Part print with two shaded views. Sizes in mm from the minimum x, y, z corner. A direction names the side the tool comes from. Coordinates: 2 decimals unless noted, no trailing zeros. Write each loop counter-clockwise with the first axis right and the second up, starting at its lowest first coordinate (ties: lowest second). Pieces come first, ordered by that corner, then holes. Notation, with made-up numbers: (-1.75, 62) - (33.25, 62) arc R34 ccw to (33.25, 99) - close; hole circle Ø1 at (18, 77.25). An arc over 180 degrees is marked (long way). Answer in a Markdown table with one row per item. Add a question column.
Q1. Pin check, flat tips, straight feed: pin 1 (1 mm diameter, centred on y = 38.5, z = 2, fed in from -X); pin 2 (3 mm diameter, centred on y = 41.5, z = 9.5, fed in from +X); pin 3 (2 mm diameter, centred on x = 39, z = 6.5, fed in from +Y). Stop position of each tip, or through.
Q2. Two-plate mould, pull along X, no slides. Class the marked faces 3, 4 and 5: +X half, -X half, draft (parallel to the pull), parting line (faces both ways), or undercut.
Q3. Band-saw the part on A-A (y = 26). List the corners of the cut face in (x, z).
Q4. Band-saw the part on D-D (y = 46.5). List the corners of the cut face in (x, z), and give its area (3 significant figures).
Q5. Drill centre lines: line 1 along Z through (x, y) = (23, 49); line 2 along X through (y, z) = (25, 3.25); line 3 along Z through (x, y) = (24, 47). Where is each one in solid material? Low to high. Write a range as from..to.
Q6. Band-saw the part on C-C (z = 2.25). List the corners of the cut face in (x, y), and give its area (3 significant figures).
Q7. 3-axis set-ups, long thin cutter, end or side, ignore diameter. For the marked faces 1 and 2: which of +Z, -Z, +X, -X, +Y, -Y reach the whole face in a straight line?
Q8. Band-saw the part on B-B (x = 23). List the corners of the cut face in (y, z), and give its area (3 significant figures).
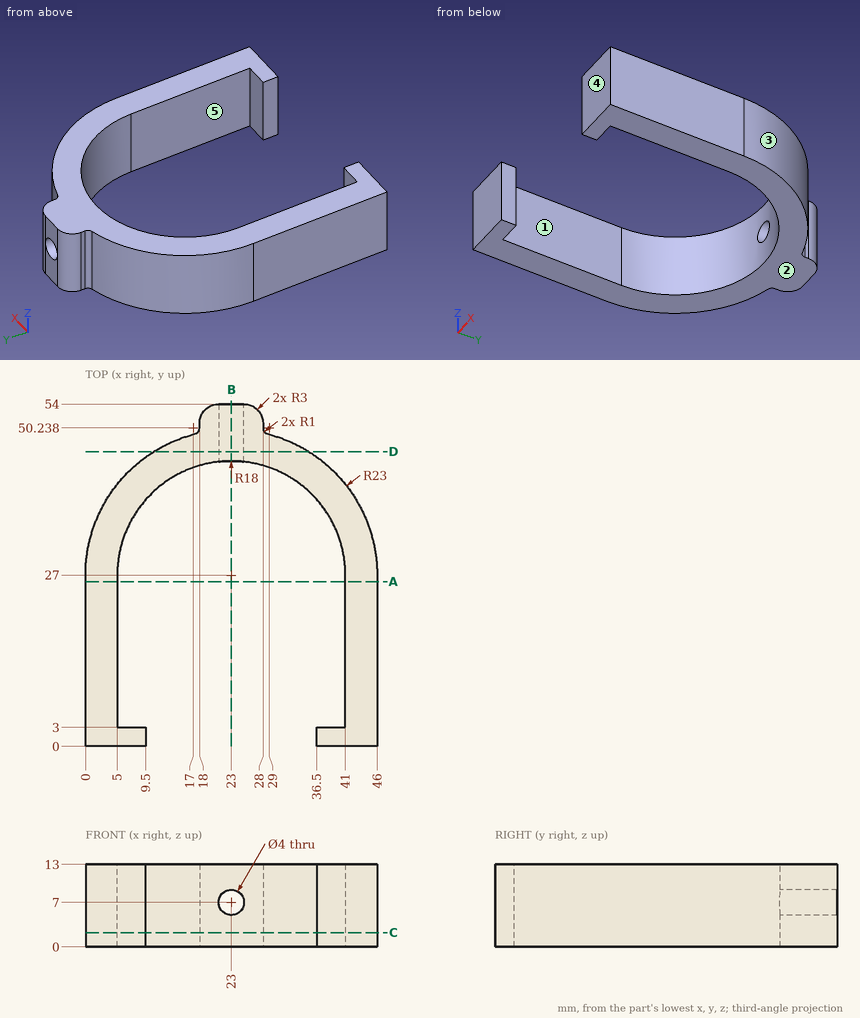
Checked values:
| question | item | result |
|---|---|---|
| 1 | pin 1 | stops at x = 2.8 |
| 1 | pin 2 | stops at x = 41.97 |
| 1 | pin 3 | stops at y = 44.44 |
| 2 | face 3 | +X half |
| 2 | face 4 | draft |
| 2 | face 5 | undercut |
| 3 | outline | (0, 0) - (5, 0) - (5, 13) - (0, 13) - close; (41, 0) - (46, 0) - (46, 13) - (41, 13) - close |
| 4 | outline | (10.8, 0) - (35.2, 0) - (35.2, 13) - (10.8, 13) - close; hole circle Ø4 at (23, 7) |
| 4 | area | 305 mm² |
| 5 | line 1 | z = 0..5, 9..13 |
| 5 | line 2 | x = 0..5, 41..46 |
| 5 | line 3 | z = 0..5.27, 8.73..13 |
| 6 | outline | (0, 0) - (9.5, 0) - (9.5, 3) - (5, 3) - (5, 27) arc R18 cw to (41, 27) - (41, 3) - (36.5, 3) - (36.5, 0) - (46, 0) - (46, 27) arc R23 ccw to (28.75, 49.27) arc R1 cw to (28, 50.24) - (28, 51) arc R3 ccw to (25, 54) - (21, 54) arc R3 ccw to (18, 51) - (18, 50.24) arc R1 cw to (17.25, 49.27) arc R23 ccw to (0, 27) - close |
| 6 | area | 657 mm² |
| 7 | face 1 | +Z, -Z |
| 7 | face 2 | -Z, +X, -X, +Y, -Y |
| 8 | outline | (45, 0) - (54, 0) - (54, 5) - (45, 5) - close; (45, 9) - (54, 9) - (54, 13) - (45, 13) - close |
| 8 | area | 81.0 mm² |
